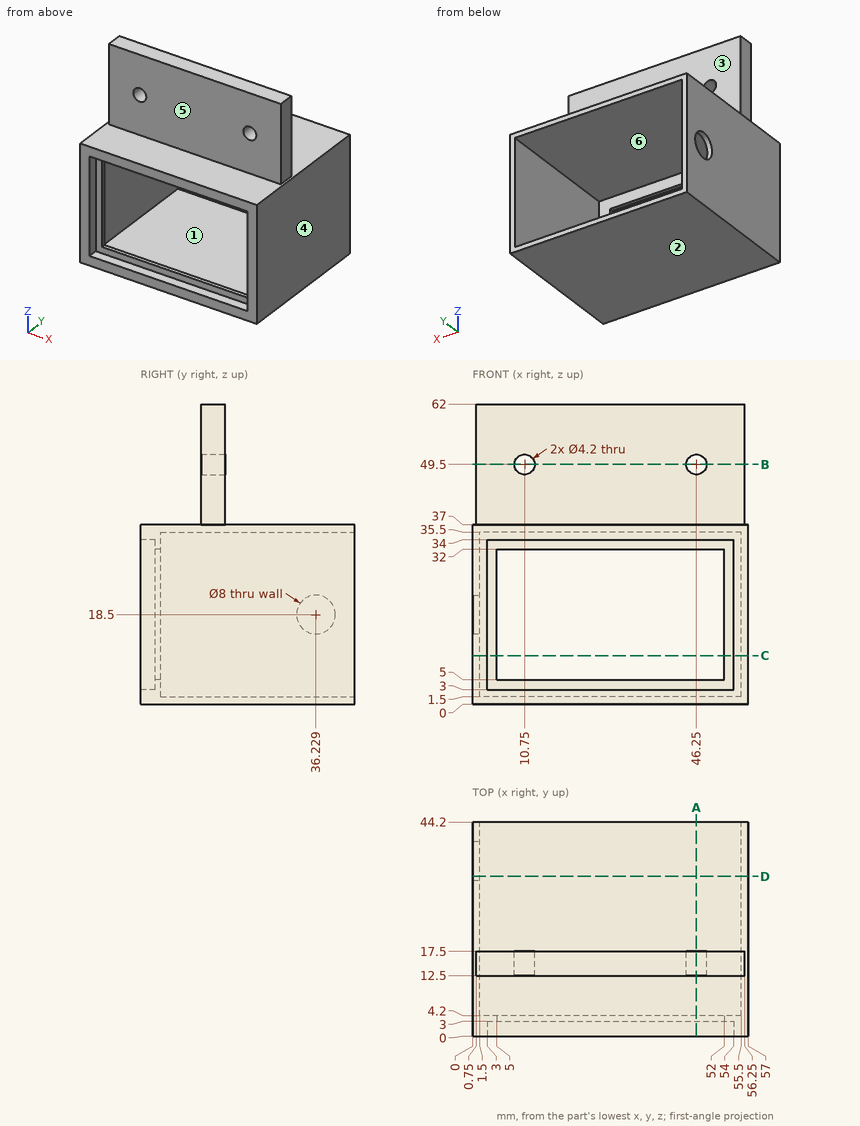
Study the drawing (mm; zero at the part's minimum x, y, z) and answer. A direction names the side the tool comes from. Give positions to 0.01 mm unless a question says otherwise; leave off trailing zeros. Write each loop counter-clockwise with the first axis right and the second up, starting at its lowest first coordinate (ties: lowest second). Pieces come first, ordered by that corner, then holes.
(1) The part is cut by section C-C on z = 10. Write down the section's boundary in (x, y), plus the area to 3 significant figures.
Final values:
outline: (0, 0) - (3, 0) - (3, 3) - (5, 3) - (5, 4.2) - (1.5, 4.2) - (1.5, 44.2) - (0, 44.2) - close; (52, 3) - (54, 3) - (54, 0) - (57, 0) - (57, 44.2) - (55.5, 44.2) - (55.5, 4.2) - (52, 4.2) - close
area: 150 mm2
(2) The part is cut by section A-A on x = 46.25. Write down the section's boundary in (y, z).
Final values:
outline: (0, 0) - (44.2, 0) - (44.2, 1.5) - (4.2, 1.5) - (4.2, 5) - (3, 5) - (3, 3) - (0, 3) - close; (0, 34) - (3, 34) - (3, 32) - (4.2, 32) - (4.2, 35.5) - (44.2, 35.5) - (44.2, 37) - (17.5, 37) - (17.5, 47.4) - (12.5, 47.4) - (12.5, 37) - (0, 37) - close; (12.5, 51.6) - (17.5, 51.6) - (17.5, 62) - (12.5, 62) - close
(3) Which of the six approach directions +Z, -Z, +X, -X, +Y, -Y give full straight-line access (tool end or side, diameter ignored) to the marked faces 1, 2 and 3?
Final values:
face 1: +Y
face 2: -Z, +X, -X, +Y, -Y
face 3: +Z, +X, -X, +Y
(4) Straight lines are drawn through the part: line 1 (Z direction, x = 46, y = 15) (3 decimals); line 2 (Z direction, x = 46.5, y = 6); line 3 (X direction, y = 26, z = 28.5). For each, find the intervals that lie inside material, in ascending order.
Final values:
line 1: z = 0 to 1.5, 35.5 to 47.415, 51.585 to 62
line 2: z = 0 to 1.5, 35.5 to 37
line 3: x = 0 to 1.5, 55.5 to 57
(5) The part is cut by section B-B on z = 49.5. Write down the section's boundary in (x, y), plus the area to 4 significant figures.
Final values:
outline: (0.75, 12.5) - (8.65, 12.5) - (8.65, 17.5) - (0.75, 17.5) - close; (12.85, 12.5) - (44.15, 12.5) - (44.15, 17.5) - (12.85, 17.5) - close; (48.35, 12.5) - (56.25, 12.5) - (56.25, 17.5) - (48.35, 17.5) - close
area: 235.5 mm2
(6) Flat-ended cylindrical pins translate along their axes: pin 1 Ø4 at (y, z) = (15, 47.5) entering from +X; pin 2 Ø4 at (y, z) = (15.5, 54.5) entering from -X; pin 3 Ø1.3 at (x, y) = (22.5, 4) entering from +Z. Find the tip coordinate at first contact, or state that the pin passes through.
Final values:
pin 1: stops at x = 56.25
pin 2: stops at x = 0.75
pin 3: stops at z = 37
(7) The mould has two halves that part along X. Classify the marked faces 4, 5 and 6: pulls with the +X half, pulls with the -X half, needs draft (parallel to the pull), parting line crosses it, or undercut.
Final values:
face 4: pulls with the +X half
face 5: needs draft
face 6: undercut
(8) The part is cut by section D-D on y = 33. Write down the section's boundary in (x, z), plus the area to 3 significant figures.
Final values:
outline: (0, 0) - (57, 0) - (57, 37) - (0, 37) - (0, 20.86) - (1.5, 20.86) - (1.5, 35.5) - (55.5, 35.5) - (55.5, 1.5) - (1.5, 1.5) - (1.5, 16.14) - (0, 16.14) - close
area: 266 mm2
